Input: part model. Units: mm. Frame: model coordinates. Round coordinates to 2 decimals unless told otherwise and drop trailing zeros. Loops run counter-clockwise (first coordinate to the right, second up) from the corner with the lowest first, then second, coordinate; pieces in that order, holes last. Notation, with made-up numbers: M -18.75,5 L 10.25,5 A31 cw 10.25,30 Z; hole C 27.5,3.25 d9. An arc over 180 degrees is marked long. Return JSON: item names as keys, results as strings. Group by question number.
1) Contact query for flat-ended pins moving along their axis: P1, Ø12, axis at x = 108, z = 7.5, coming from the -Y side; P2, Ø8.5, axis at x = 29.5, y = 77.5, coming from the +Z side; P3, Ø7, axis at x = 77, y = 179.5, coming from the -Z side. Output: stop coordinate, or through.
2) Section C-C (y = 55). Output: boundary loops of the cut face in (x, z).
3) Material intervals for line 1 (X direction, y = 325.6, z = -16.5); line 2 (Z direction, x = 85.5, y = 169.5); line 3 (Y direction, x = 78.5, z = 3.5), sorted ascending. Write a range as from..to.
4) Section B-B (z = -11.5). Output: boundary loops of the cut face in (x, y), plus the area to 3 significant figures.
5) Section A-A (y = 111.5). Output: boundary loops of the cut face in (x, z).
from build123d import *

# Parameters (mm, degrees)
BOSS_EXTRU_1_DEPTH           = 9
ESQUISSE36_W                 = 5
ESQUISSE36_H                 = 5
ESQUISSE36_H_2               = 15
BOSS_EXTRU_4_DEPTH           = 8
BALAYAGE2_PROFILE_R          = 2.5
BALAYAGE3_PROFILE_R          = 2.5
CONG_2_R                     = 30
CONG_3_R                     = 10
BALAYAGE4_PROFILE_R          = 2.5
ENL_V_MAT_EXTRU_2_DEPTH      = 363.063201398
ENL_V_MAT_EXTRU_2_DEPTH_BACK = 10
ESQUISSE103_R                = 1.5


with BuildPart() as part:
    # Esquisse1 → Boss.-Extru.1 (new body)
    with BuildSketch(Plane.XY):
        Polygon((0, 0), (90, 195), (140, 235), (150.932632942, 235), (132.339381175, 195.201149163), (127.997155304, 127.139031538), (76.950468366, 0), align=None)
    extrude(amount=BOSS_EXTRU_1_DEPTH)

    # Esquisse36 → Boss.-Extru.4 (add)
    with BuildSketch(Plane(origin=(0, 0, 0), x_dir=(0, 0, 1), z_dir=(-0.9079593845004518, 0.4190581774617469, 0))):
        with Locations((4.5, 172.267315949)):
            Rectangle(ESQUISSE36_W, ESQUISSE36_H)
        with Locations((4.5, 82.267315949)):
            Rectangle(ESQUISSE36_W, ESQUISSE36_H)
        with Locations((4.5, 197.267315949)):
            Rectangle(ESQUISSE36_W, ESQUISSE36_H_2)
    extrude(amount=BOSS_EXTRU_4_DEPTH)

    # Balayage2: sweep along a path in Esquisse37
    with BuildLine(Plane(origin=(-7.263675076, 3.35246542, 0), x_dir=(0, 0, 1), z_dir=(-0.9079593845004523, 0.4190581774617459, 0))) as balayage2_path:
        Line((4.5, 354.767315949), (4.5, 154.767315949))
    # Balayage2 profile (on start of the path) → Balayage2 (sweep)
    with BuildSketch(Plane(origin=(141.404469769, 325.46677925, 4.5), x_dir=(-0.9079593845004521, 0.41905817746174584, 0), z_dir=(-0.4190581774617459, -0.9079593845004523, 0))):
        Circle(BALAYAGE2_PROFILE_R)
    sweep(path=balayage2_path.line)

    # Balayage3: sweep along a path in Esquisse50
    with BuildLine(Plane(origin=(-7.263675076, 3.35246542, 0), x_dir=(0, 0, 1), z_dir=(-0.9079593845004512, 0.41905817746174806, 0))) as balayage3_path:
        Line((4.5, 84.767315949), (4.5, 64.767315949))
    # Balayage3 profile (on start of the path) → Balayage3 (sweep)
    with BuildSketch(Plane(origin=(28.258761854, 80.317745435, 4.5), x_dir=(-0.9079593845004512, 0.41905817746174806, 0), z_dir=(-0.41905817746174806, -0.9079593845004512, 0))):
        Circle(BALAYAGE3_PROFILE_R)
    sweep(path=balayage3_path.line)

    # Congé2
    cong_2_edges = [part.edges().sort_by_distance(p)[0] for p in [
        (90, 195, 4.5),
        (140, 235, 4.5),
        (132.339381175, 195.201149163, 4.5),
        (127.997155304, 127.139031538, 4.5),
        (76.950468366, 0, 4.5),
    ]]
    fillet(cong_2_edges, radius=CONG_2_R)

    # Congé3
    # the kernel refuses this fillet: 10 mm, written as the material it takes off along each edge
    with BuildSketch(Plane(origin=(150.932632942, 235, -7.177129448), x_dir=(-1, 0, 0), z_dir=(0, 0, 1))) as cong_3_piece_1:
        with BuildLine():
            CenterArc((10.275185308, -1.631673015), CONG_3_R, 154.958930111, 15.650284086)
            Line((1.215139114, 2.601004974), (0, 0))
            Line((0, 0), (0.409201162, 0))
        make_face()
    extrude(amount=23.354258897, mode=Mode.SUBTRACT)

    # Balayage4: sweep along a path in Esquisse88
    with BuildLine(Plane(origin=(148.668144845, 322.11431383, 0), x_dir=(0.907959384500452, -0.4190581774617463, 0), z_dir=(0.41905817746174623, 0.9079593845004519, 0))) as balayage4_path:
        Line((-8, 20.5), (-8, -29.5))
    # Balayage4 profile (on start of the path) → Balayage4 (sweep)
    with BuildSketch(Plane(origin=(141.404469769, 325.46677925, -20.5), x_dir=(0, 1, 0), z_dir=(0, 0, 1))):
        Circle(BALAYAGE4_PROFILE_R)
    sweep(path=balayage4_path.line)

    # Esquisse103 → Enlèv. mat.-Extru.2 (cut, two sides: drawn at the far end of the back side and taken through both)
    with BuildSketch(Plane(origin=(0, 0, 0), x_dir=(1, 0, 0), z_dir=(0, 1, 0)).offset(-ENL_V_MAT_EXTRU_2_DEPTH_BACK)):
        with Locations(Location((141.404469769, 16.5, 0), (0, 0, 90))):
            Circle(ESQUISSE103_R)
        with Locations(Location((141.391933609, -25.5, 0), (0, 0, 90))):
            Circle(ESQUISSE103_R)
    extrude(amount=ENL_V_MAT_EXTRU_2_DEPTH + ENL_V_MAT_EXTRU_2_DEPTH_BACK, mode=Mode.SUBTRACT)


solid = part.part
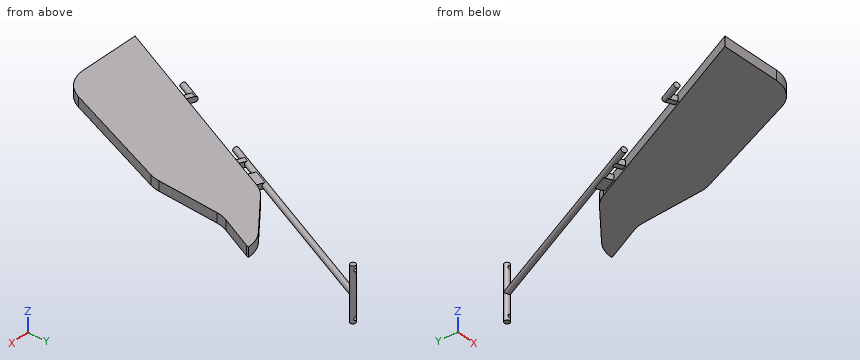
Returned:
{
 "1": {"P1": "stops at y = 62.39", "P2": "stops at z = 7", "P3": "stops at z = 2"},
 "2": {"outline": "M 25.38,0 L 99.03,0 L 99.03,9 L 25.38,9 Z"},
 "3": {"line 1": "x = 138.91..139.9, 142.9..143.9", "line 2": "z = 0..9", "line 3": "y = 9.42..170.08, 172.77..194.64"},
 "4": {"outline": "C 141.4,325.47 d5", "area": "19.6 mm^2"},
 "5": {"outline": "M 51.46,0 L 121.72,0 L 121.72,9 L 51.46,9 Z"}
}
